from build123d import *

# Parameters (mm, degrees)
SKETCH_1_R                     = 40
EXTRUDE_1_DEPTH                = 40
SKETCH_3_R                     = 30
CUT_EXTRUDE_2_DEPTH            = 35
HOLE_WIZARD_21_5_21_5_1_REACH  = 100.524
HOLE_WIZARD_21_5_21_5_1_BORE_R = 10.75


with BuildPart() as part:
    # 草圖1 → 填料-伸長1 (new body)
    with BuildSketch(Plane(origin=(0, 0, 0), x_dir=(1, 0, 0), z_dir=(0, 1, 0))):
        with Locations(Location((0, 0, 0), (0, 0, 270))):
            Circle(SKETCH_1_R)
    extrude(amount=EXTRUDE_1_DEPTH)

    # 草圖3 → 除料-伸長2 (cut)
    with BuildSketch(Plane(origin=(0, 40, 0), x_dir=(1, 0, 0), z_dir=(0, 1, 0))):
        with Locations(Location((0, 0, 0), (0, 0, 270))):
            Circle(SKETCH_3_R)
    extrude(amount=-CUT_EXTRUDE_2_DEPTH, mode=Mode.SUBTRACT)

    # Ø21.5 (21.5) 直徑孔1 bore (on position points) → Ø21.5 (21.5) 直徑孔1 (cut, up to next)
    with BuildSketch(Plane(origin=(-21.744758151, 21.94181737, 33.573285406), x_dir=(0.839332135156, 0, 0.543618953768), z_dir=(-0.543618953768, 0, 0.839332135156)), mode=Mode.PRIVATE) as hole_wizard_21_5_21_5_1_sk1:
        Circle(HOLE_WIZARD_21_5_21_5_1_BORE_R)
    hole_wizard_21_5_21_5_1_tool1 = extrude(hole_wizard_21_5_21_5_1_sk1.sketch, amount=-HOLE_WIZARD_21_5_21_5_1_REACH, mode=Mode.PRIVATE) & part.part
    add(hole_wizard_21_5_21_5_1_tool1.solids().sort_by_distance((-21.744758, 21.941817, 33.573285))[0], mode=Mode.SUBTRACT)


solid = part.part
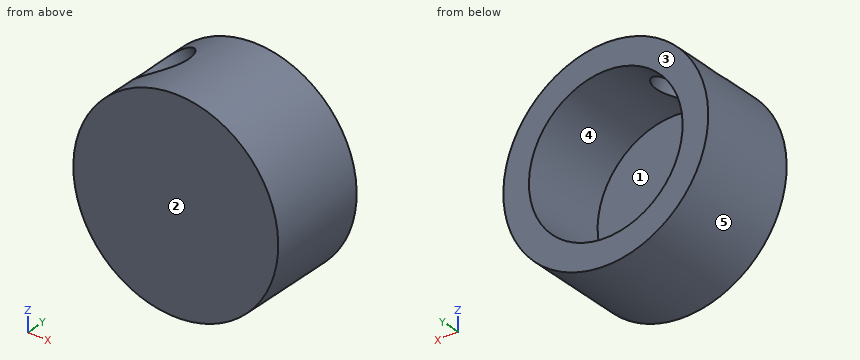
Part model, mm, in its own coordinate system. Face numbers are marked on the shaded views. A direction names the side the tool comes from. Round coordinates to 2 decimals unless told otherwise and drop trailing zeros. Loops run counter-clockwise (first coordinate to the right, second up) from the corner with the lowest first, then second, coordinate; pieces in that order, holes last. Notation, with made-up numbers: (-33, 55) - (0, 55) arc R12 ccw to (0, 76) - close; hole circle Ø5 at (13.5, 75.5). An arc over 180 degrees is marked (long way). Answer as a JSON object with one key per item and string values.
Item 1: Band-saw the part on B-B on x = 24. List the corners of the cut face in (y, z), plus the area to 3 significant figures.
Output:
{"outline": "(0, -32) - (40, -32) - (40, -18) - (5, -18) - (5, 18) - (40, 18) - (40, 32) - (0, 32) - close", "area": "1,300 mm2"}
Item 2: Band-saw the part on A-A on z = 0. List the corners of the cut face in (x, y), plus the area to 3 significant figures.
Output:
{"outline": "(-40, 0) - (40, 0) - (40, 40) - (30, 40) - (30, 5) - (-30, 5) - (-30, 40) - (-40, 40) - close", "area": "1,100 mm2"}
Item 3: Wall check: L1, parallel to X at y = 19.5, z = 0; L2, parallel to Y at x = -17.5, z = -20; L3, parallel to X at y = 13, z = 25.5. Give the ranges that are in metal, low to high.
Output:
{"L1": "-40 to -30, 30 to 40", "L2": "0 to 5", "L3": "-30.82 to -23.63, 15.8 to 30.82"}
Item 4: Tool access for the marked faces 1 and 2: list every direction of +Z, -Z, +X, -X, +Y, -Y with a clear straight run to the whole face (end or side of a thin tool).
Output:
{"face 1": "+Y", "face 2": "+Z, -Z, +X, -X, -Y"}
Item 5: Pull direction Z, two halves, no side cores. Call the marked faces 3, 4 and 5: pulls with the +Z half, pulls with the -Z half, needs draft (parallel to the pull), parting line crosses it, or undercut.
Output:
{"face 3": "needs draft", "face 4": "undercut", "face 5": "parting line crosses it"}
Item 6: Band-saw the part on C-C on y = 36.5. List the corners of the cut face in (x, z).
Output:
{"outline": "circle Ø80 at (0, 0); hole circle Ø60 at (0, 0)"}
Item 7: Band-saw the part on D-D on z = -32. List the corners of the cut face in (x, y), plus the area to 3 significant figures.
Output:
{"outline": "(-24, 0) - (24, 0) - (24, 40) - (-24, 40) - close", "area": "1,920 mm2"}
Item 8: Pin check, flat tips, straight feed: pin 1 (3 mm diameter, centred on y = 20, z = -25, fed in from +X); pin 2 (10 mm diameter, centred on y = 18, z = 17, fed in from +X); pin 3 (10 mm diameter, centred on y = 14, z = 3, fed in from +X). Stop position of each tip, or through.
Output:
{"pin 1": "x = 32.37", "pin 2": "x = 38.16", "pin 3": "x = 40"}
